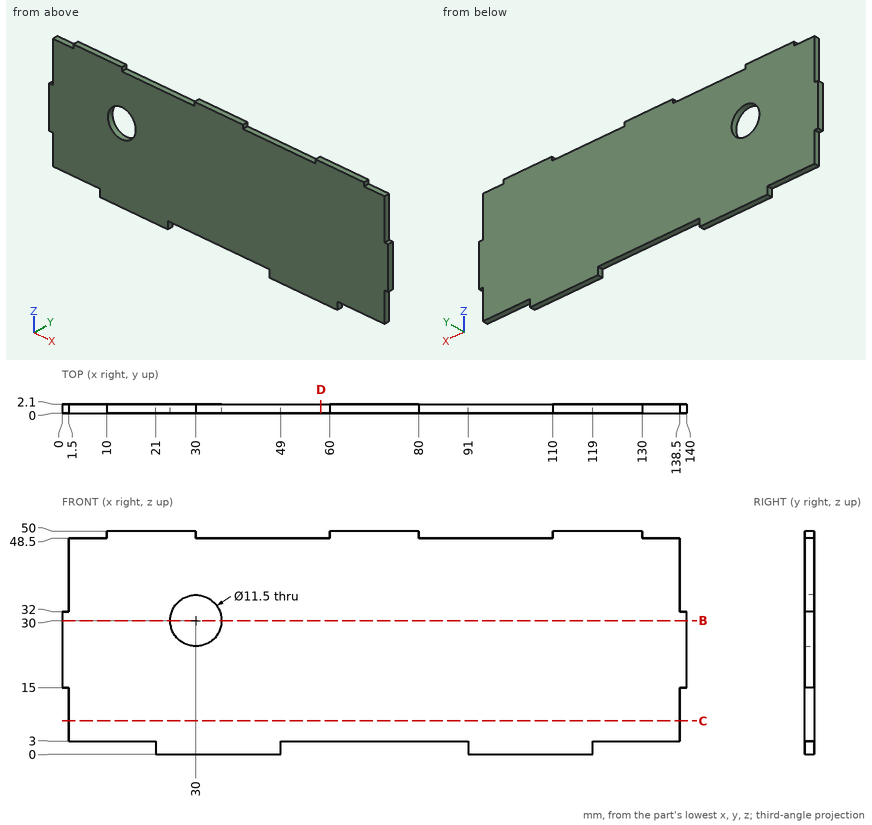
Geometry check sheet. Reference: drawing and pictorial views, mm from the part's lowest x, y, z. Round coordinates to 2 decimals unless told otherwise and drop trailing zeros. Order: outer loops, then holes, each group sorted by start corner. A loop starts at its lowest first (then second) coordinate and runs counter-clockwise, first axis right, second up. Notation, with made-up numbers: (48.25, 8.5) - (54.25, 8.5) arc R18 cw to (54.25, 25.5) - close; hole circle Ø10 at (-15.75, -12.5). An arc over 180 degrees is marked (long way). Use a Markdown table: item, result. Add a question column.
1) Gauge pin test, flat ends, axial feed: P1, Ø0.6, axis at y = 1.5, z = 39.5, coming from the +X side; P2, Ø1, axis at x = 126.5, y = 1, coming from the -Z side; P3, Ø1, axis at y = 1, z = 8.5, coming from the -X side. Record the tip position at first contact, or that the pin passes through.
2) Section check C-C (z = 7.5). Record the cut outline in (x, y).
3) Section check B-B (z = 30). Record the cut outline in (x, y).
4) Section check D-D (x = 58). Record the cut outline in (y, z).
5) Thickness scan on line 1 along X through (y, z) = (1.1, 30); line 2 along X through (y, z) = (1.9, 2); line 3 along X through (y, z) = (0.4, 37). Record the ranges inside material, lowest first.
Established:
| question | item | result |
|---|---|---|
| 1 | P1 | x = 138.5 |
| 1 | P2 | z = 3 |
| 1 | P3 | x = 1.5 |
| 2 | outline | (1.5, 0) - (138.5, 0) - (138.5, 2.1) - (1.5, 2.1) - close |
| 3 | outline | (0, 0) - (24.25, 0) - (24.25, 2.1) - (0, 2.1) - close; (35.75, 0) - (140, 0) - (140, 2.1) - (35.75, 2.1) - close |
| 4 | outline | (0, 3) - (2.1, 3) - (2.1, 48.5) - (0, 48.5) - close |
| 5 | line 1 | 0 to 24.25, 35.75 to 140 |
| 5 | line 2 | 21 to 49, 91 to 119 |
| 5 | line 3 | 1.5 to 138.5 |
